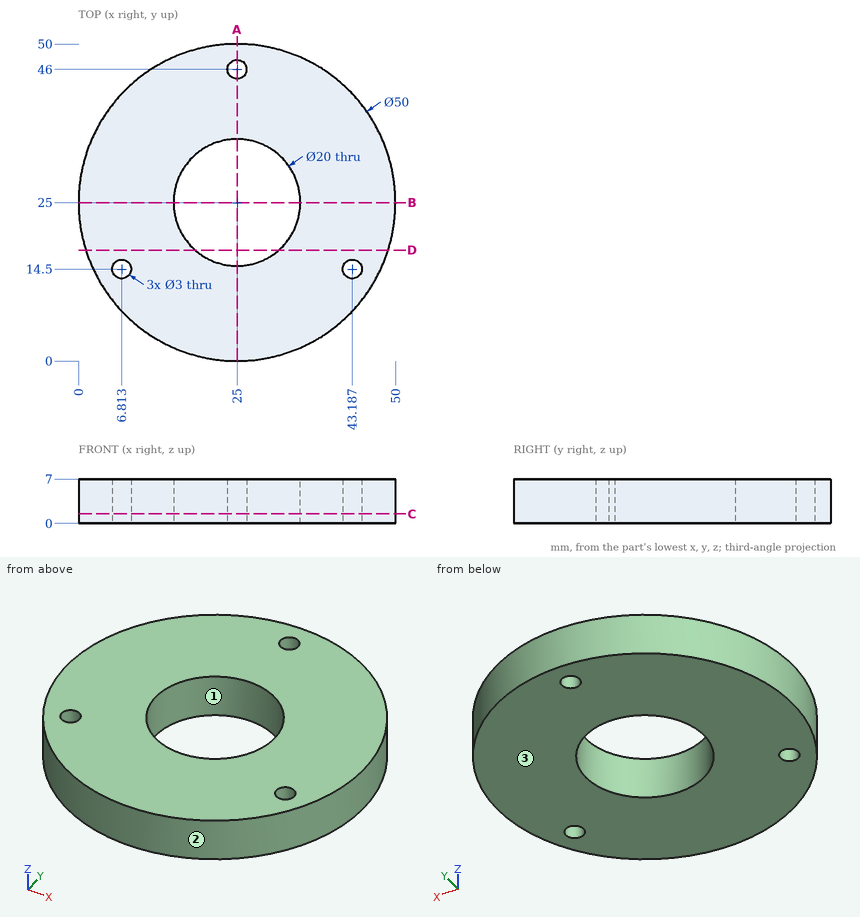
Design review of the part shown in the three views and the two pictorial views. Dimensions are in mm from the part's minimum x, y and z. Round coordinates to 2 decimals unless told otherwise and drop trailing zeros. Loops run counter-clockwise (first coordinate to the right, second up) from the corner with the lowest first, then second, coordinate; pieces in that order, holes last.
1) Consider section B-B on y = 25. State the section outline as (x, z) points, then the cut area to 3 significant figures.
Values follow:
outline: (0, 0) - (15, 0) - (15, 7) - (0, 7) - close; (35, 0) - (50, 0) - (50, 7) - (35, 7) - close
area: 210 mm2
2) Consider section C-C on z = 1.5. State the section outline as (x, y) points.
Values follow:
outline: circle Ø50 at (25, 25); hole circle Ø3 at (6.81, 14.5); hole circle Ø20 at (25, 25); hole circle Ø3 at (25, 46); hole circle Ø3 at (43.19, 14.5)
3) Wall thickness on line 1 along Y through (x, z) = (25, 5.25); line 2 along Y through (x, z) = (16.5, 4.5) (1 decimal); line 3 along X through (y, z) = (26, 1.75): over which ranges is each line inside the solid? List them lowest first.
Values follow:
line 1: y = 0 to 15, 35 to 44.5, 47.5 to 50
line 2: y = 1.5 to 19.7, 30.3 to 48.5
line 3: x = 0.02 to 15.05, 34.95 to 49.98
4) Consider section D-D on y = 17.5. State the section outline as (x, z) points (1 decimal).
Values follow:
outline: (1.2, 0) - (18.4, 0) - (18.4, 7) - (1.2, 7) - close; (31.6, 0) - (48.8, 0) - (48.8, 7) - (31.6, 7) - close
5) The part is to be moulded in two halves that separate along X. For the marked faces 1, 2 and 3, say which applies: pulls with the +X half, pulls with the -X half, needs draft (parallel to the pull), parting line crosses it, or undercut.
Values follow:
face 1: undercut
face 2: parting line crosses it
face 3: needs draft
6) Consider section A-A on x = 25. State the section outline as (y, z) points, then the cut area to 3 significant figures.
Values follow:
outline: (0, 0) - (15, 0) - (15, 7) - (0, 7) - close; (35, 0) - (44.5, 0) - (44.5, 7) - (35, 7) - close; (47.5, 0) - (50, 0) - (50, 7) - (47.5, 7) - close
area: 189 mm2
7) Clearance check with flat-ended pins moving along their axes: P1, Ø2, axis at x = 9, y = 30.5, coming from the -Z side; P2, Ø2.5, axis at x = 6.81, y = 14.5, coming from the -Z side; P3, Ø3, axis at y = 33.5, z = 3.5, coming from the +X side; P4, Ø4, axis at x = 34, z = 4, coming from the +Y side. State where each tip first meets the part, or that it passes through.
Values follow:
P1: stops at z = 0
P2: passes through
P3: stops at x = 49
P4: stops at y = 49
